Work out the finished part from the listing and answer in its coordinate system (mm). Face numbers are marked on the shaded views. A direction names the side the tool comes from. Give positions to 0.01 mm unless a question says otherwise; leave off trailing zeros. Order: outer loops, then holes, each group sorted by start corner. A loop starts at its lowest first (then second) coordinate and runs counter-clockwise, first axis right, second up. Notation, with made-up numbers: (26, -31.75) - (73, -31.75) arc R33 ccw to (73, -1.75) - close; hole circle Ø9 at (18, 24). An arc over 180 degrees is marked (long way). Return JSON: item names as keys, results as strings. Group by question number.
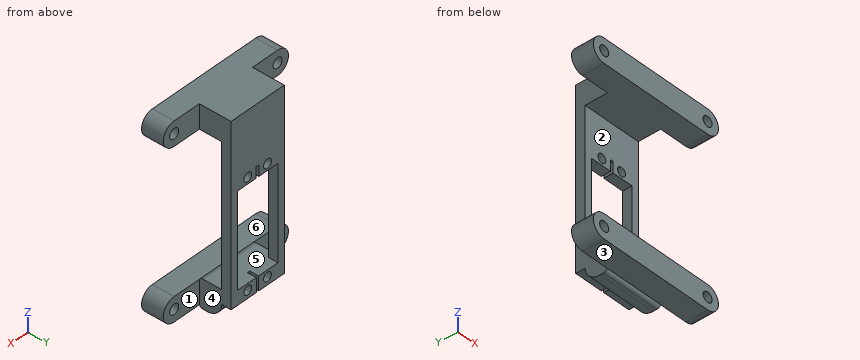
Autodesk Inventor part; units mm, degrees
ref_plane "YZ Plane" through (0, 0, 0) normal (1, 0, 0) x (0, 1, 0)
ref_plane "XZ Plane" through (0, 0, 0) normal (0, 1, 0) x (-1, 0, 0)
ref_plane "XY Plane" through (0, 0, 0) normal (0, 0, 1) x (1, 0, 0)
sketch "Sketch1" plane through (0, 0, 0) normal (0, 1, 0) x (-1, 0, 0)
  circle A0 centre (-26.1551, -3.0475) radius 2.3
  arc A1 (-34.9051, -0.0475) -> (-17.4051, -0.0475) centre (-26.1551, -0.0475) ccw
  arc A2 (17.5949, -0.0475) -> (35.0949, -0.0475) centre (26.3449, -0.0475) ccw
  circle A3 centre (26.3449, -3.0475) radius 2.3
  circle A4 centre (-26.1551, -3.0475) radius 2.3
  circle A5 centre (26.3449, -3.0475) radius 2.3
  circle A6 centre (26.3449, -0.0475) radius 8.75
  circle A7 centre (-26.1551, -0.0475) radius 8.75
  line L0 (-34.9051, -0.0475) -> (-17.4051, -0.0475)
  line L1 (17.5949, -0.0475) -> (35.0949, -0.0475)
  circle A8 centre (-26.1551, -3.0475) radius 5.5
  circle A9 centre (26.3449, -3.0475) radius 5.5
  line L2 (-26.1551, -8.5475) -> (26.3449, -8.5475)
  line L3 (-26.1551, 2.4525) -> (26.3449, 2.4525)
  point P0 (0, 0)
  dimension "d0" = 11
  dimension "d1" = 11
  dimension "d41" = 4.6
  dimension "d42" = 4.6
extrude "Extrusion1" add sketch "Sketch1" along normal blind 10 contours L2 A8 L0 A1 | A1 A7 L3 A6 A2 L2 | A7 L0 A8 L3 | A8 L0 | L0 A8 | A2 L1 A9 L2 | L3 A9 L1 A6 | A9 L1 | A9 L1 picked at (-18.6939, -1.0014) picked at (-20.5799, 1.133) picked at (18.8536, -1.0809) picked at (20.7697, 1.133)
sketch "Sketch2" plane through (0, 10, 0) normal (0, 1, 0) x (1, 0, 0)
  line L0 (26.1551, 8.5475) -> (-26.3449, 8.5475)
  line L1 (-26.3449, -2.4525) -> (26.1551, -2.4525)
  arc A0 (-26.3449, 8.5475) -> (-26.3449, -2.4525) centre (-26.3449, 3.0475) ccw
  arc A1 (26.1551, -2.4525) -> (26.1551, 8.5475) centre (26.1551, 3.0475) ccw
  line L2 (-31.8449, 3.0475) -> (31.6551, 3.0475)
  line L3 (13.4051, -3.4525) -> (-13.5949, -3.4525)
  line L4 (-13.5949, -3.4525) -> (-13.5949, 9.5475)
  line L5 (-13.5949, 9.5475) -> (13.4051, 9.5475)
  line L6 (13.4051, 9.5475) -> (13.4051, -3.4525)
  line L7 (13.4051, -3.4525) -> (-13.5949, 9.5475) construction
  line L8 (-13.5949, -3.4525) -> (13.4051, 9.5475) construction
  point P0 (0, 0)
  point P1 (-0.0949, 3.0475)
  dimension "d4" = 27
  dimension "d5" = 13
extrude "Extrusion2" add sketch "Sketch2" along normal blind 14.56 contours L6 L2 L4 L0 | L0 L4 L5 L6 | L6 L1 L4 L2 | L6 L3 L4 L1
fillet "Fillet1" radius 2 2 edges at (-0.0949, 10, 3.4525) (-0.0949, 10, -9.5475)
sketch "Sketch3" plane through (0, 24.56, 0) normal (0, 1, 0) x (1, 0, 0)
  arc A0 (-6.3682, 1.0898) -> (-3.9766, 1.2056) centre (-5.0949, -0.4525) ccw
  arc A1 (3.6318, 1.0898) -> (6.0234, 1.2056) centre (4.9051, -0.4525) ccw
  circle A2 centre (4.9051, -0.4525) radius 2
  circle A3 centre (-5.0949, -0.4525) radius 2
  line L0 (-13.5949, 9.5475) -> (-13.5949, -3.4525)
  line L1 (13.4051, 9.5475) -> (-13.5949, 9.5475)
  line L2 (-13.5949, -3.4525) -> (13.4051, -3.4525)
  line L3 (13.4051, -3.4525) -> (13.4051, 9.5475)
  point P0 (0, 0)
  point P1 (6.0234, 1.2056)
  point P2 (3.6318, 1.0898)
  point P3 (-3.9766, 1.2056)
  point P4 (-6.3682, 1.0898)
  dimension "d12" = 8.5
  dimension "d13" = 8.5
  dimension "d43" = 2
  dimension "d44" = 2
extrude "Extrusion3" cut sketch "Sketch3" against normal blind 10 contours A3 A0 | A2 A1
sketch "Sketch4" plane through (0, 24.56, 0) normal (0, 1, 0) x (1, 0, 0)
  line L0 (13.4051, 9.5475) -> (-13.5949, 9.5475)
  line L1 (-13.5949, -2.4525) -> (-13.5949, 8.5475)
  line L2 (13.4051, 9.5475) -> (-13.5949, 9.5475)
  line L3 (-13.5949, 9.5475) -> (-13.5949, 3.0475)
  line L4 (-13.5949, 3.0475) -> (13.4051, 3.0475)
  line L5 (13.4051, 3.0475) -> (13.4051, 9.5475)
  point P0 (0, 0)
extrude "Extrusion4" cut sketch "Sketch4" against normal blind 4.2875
fillet "Fillet2" radius 6.7625 1 edges at (-0.0949, 20.2725, -9.5475)
sketch "Sketch5" plane through (0, 24.56, 0) normal (0, 1, 0) x (1, 0, 0)
  line L0 (-13.5949, -3.4525) -> (13.4051, -3.4525)
  line L1 (-10.3949, -3.4525) -> (-10.3949, -67.4525)
  line L2 (10.2051, -3.4525) -> (10.2051, -67.4525)
  line L3 (-13.5949, 3.0475) -> (-13.5949, -3.4525)
  circle A0 centre (-5.0949, -49.4525) radius 2
  line L4 (13.4051, -3.4525) -> (13.4051, 3.0475)
  circle A1 centre (4.9051, -49.4525) radius 2
  circle A2 centre (4.9051, -49.4525) radius 3
  circle A3 centre (-5.0949, -49.4525) radius 3
  line L5 (-10.3949, -67.4525) -> (10.2051, -67.4525)
  line L6 (-10.3949, -67.4525) -> (-13.5949, -67.4525)
  line L7 (-13.5949, -67.4525) -> (-13.5949, -3.4525)
  line L8 (10.2051, -67.4525) -> (13.4051, -67.4525)
  line L9 (13.4051, -67.4525) -> (13.4051, -3.4525)
  line L10 (-5.0949, -46.4525) -> (4.9051, -46.4525)
  line L11 (10.2051, -46.4525) -> (-10.3949, -46.4525)
  line L12 (-0.65, -46.4525) -> (-0.65, -51.4525)
  line L13 (-0.65, -51.4525) -> (0.65, -51.4525)
  line L14 (0.65, -51.4525) -> (0.65, -46.4525)
  line L15 (0, -46.4525) -> (-0.65, -51.4525) construction
  line L16 (0, -46.4525) -> (0.65, -51.4525) construction
  point P0 (0, 0)
  point P1 (13.4051, -0.2025)
  point P2 (4.9051, -46.4525)
  dimension "d28" = 6
  dimension "d29" = 6
  dimension "d19" = 3.2
  dimension "d20" = 64
  dimension "d21" = 3.2
  dimension "d22" = 64
  dimension "d23" = 46
  dimension "d24" = 8.5
  dimension "d25" = 4
  dimension "d26" = 8.5
  dimension "d27" = 4
  dimension "d30" = 1.3
extrude "Extrusion5" add sketch "Sketch5" against normal blind 4.2875 contours L0 L1 L6 L7 | L0 L9 L8 L2 | A2 | A3 | L11 L10 L12 L13 L14 L2 L5 L1
sketch "Sketch6" plane through (0, 24.56, 0) normal (0, 1, 0) x (1, 0, 0)
  line L0 (13.4051, -67.4525) -> (-13.5949, -67.4525)
  line L1 (-13.5949, -67.4525) -> (13.4051, -67.4525)
  line L2 (13.4051, -67.4525) -> (13.4051, -78.4525)
  line L3 (13.4051, -78.4525) -> (-13.5949, -78.4525)
  line L4 (-13.5949, -78.4525) -> (-13.5949, -67.4525)
  circle A0 centre (26.1551, 3.0475) radius 2.3
  circle A1 centre (-26.3449, 3.0475) radius 2.3
  point P0 (0, 0)
  dimension "d34" = 11
extrude "Extrusion6" add sketch "Sketch6" against normal up to surface (14.56 mm away) contours L2 L3 L4 L0
ref_plane "Work Plane1" through (-13.5949, 24.56, 34.9525) normal (0, 0, 1) x (1, 0, 0)
sketch "Sketch7" plane through (0, 24.56, 0) normal (0, 1, 0) x (1, 0, 0)
  point P0 (0, 0)
mirror "Mirror1" about plane through (-13.5949, 24.56, 34.9525) normal (0, 0, 1) of "Extrusion1"
sketch "Sketch8" plane through (0, 24.56, 0) normal (0, 1, 0) x (1, 0, 0)
  line L0 (0.6, -3.9565) -> (-0.6, -3.9565)
  line L1 (-0.6, -3.9565) -> (-0.6, 3.9565)
  line L2 (-0.6, 3.9565) -> (0.6, 3.9565)
  line L3 (0.6, 3.9565) -> (0.6, -3.9565)
  line L4 (0.6, -3.9565) -> (-0.6, 3.9565) construction
  line L5 (-0.6, -3.9565) -> (0.6, 3.9565) construction
  point P0 (0, 0)
  dimension "d38" = 1.2
extrude "Extrusion7" cut sketch "Sketch8" against normal blind 4
properties part number "SERVO_MOUNT_TOBASE"
1. Each of these flat-tipped pins is pushed along its axis until it touches: pin 1 (6.5 mm diameter, centred on x = -5.09, z = 49.45, fed in from -Y); pin 2 (1.2 mm diameter, centred on x = 5, z = 0.5, fed in from +Y); pin 3 (4.5 mm diameter, centred on x = 4, y = 23, fed in from -Z). Where does it stop, or does it pass through?
2. The part is cut by section A-A (z = 26.5). Give the vertices of the cut face in (x, y).
3. The part is cut by section C-C (z = 50.5). Give the vertices of the cut face in (x, y).
4. A tool of negligible diameter and unlimited length cuts with its end or side. For the marked faces 4, 5 and 6, from which of +Z, -Z, +X, -X, +Y, -Y can it reach the whole face along a straight path? Write none if from no direction.
5. The part is cut by section D-D (y = 4). Give the vertices of the cut face in (x, z), and give its area (3 significant figures).
6. Determine the mould class of the marked faces 1, 2 and 3 for opening direction Z: released by +Z, released by -Z, zero draft, split by the parting line, or undercut.
7. The part is cut by section B-B (x = 15). Give the vertices of the cut face in (y, z), and give its area (3 significant figures).
8. Consider probe 1 along Z at (x, y) = (28, 7.75); probe 2 along X at (y, z) = (16.75, -1); probe 3 along Z at (x, y) = (8.5, 13.25). Determine where each line is inside the solid, lowest interval first. Write a range as from..to.
Answers:
{
 "1": {"pin 1": "stops at y = 20.27", "pin 2": "stops at y = 14.56", "pin 3": "stops at z = -3.05"},
 "2": {"outline": "(-13.59, 20.27) - (-10.39, 20.27) - (-10.39, 24.56) - (-13.59, 24.56) - close; (10.21, 20.27) - (13.41, 20.27) - (13.41, 24.56) - (10.21, 24.56) - close"},
 "3": {"outline": "(-13.59, 20.27) - (-6.8, 20.27) - (-6.8, 24.56) - (-13.59, 24.56) - close; (-3.39, 20.27) - (-0.65, 20.27) - (-0.65, 24.56) - (-3.39, 24.56) - close; (0.65, 20.27) - (3.2, 20.27) - (3.2, 24.56) - (0.65, 24.56) - close; (6.61, 20.27) - (13.41, 20.27) - (13.41, 24.56) - (6.61, 24.56) - close"},
 "4": {"face 4": "+Z, -Z, +X, +Y", "face 5": "-Y", "face 6": "+X, -X, -Y"},
 "5": {"outline": "(-26.34, -8.55) - (26.16, -8.55) arc R5.5 ccw to (26.16, 2.45) - (-26.34, 2.45) arc R5.5 ccw to start; (-26.34, 67.45) - (26.16, 67.45) arc R5.5 ccw to (26.16, 78.45) - (-26.34, 78.45) arc R5.5 ccw to start; hole circle Ø4.6 at (-26.34, -3.05); hole circle Ø4.6 at (-26.34, 72.95); hole circle Ø4.6 at (26.16, -3.05); hole circle Ø4.6 at (26.16, 72.95)", "area": "1,280 mm^2"},
 "6": {"face 1": "zero draft", "face 2": "undercut", "face 3": "released by -Z"},
 "7": {"outline": "(0, -8.55) - (10, -8.55) - (10, 2.45) - (0, 2.45) - close; (0, 67.45) - (10, 67.45) - (10, 78.45) - (0, 78.45) - close", "area": "220 mm^2"},
 "8": {"probe 1": "z = -8.23..-4.42, -1.67..2.13, 67.77..71.58, 74.33..78.13", "probe 2": "x = -13.59..-6.47, -3.72..3.53, 6.28..13.41", "probe 3": "z = -9.55..3.45, 67.45..78.45"}
}
